```python
from build123d import *

# Parameters (mm, degrees)
SKETCH1_W           = 6.35
SKETCH1_H           = 3.0988
SKETCH1_H_2         = 25.146
BOSS_EXTRUDE1_DEPTH = 6.35


with BuildPart() as part:
    # Sketch1 → Boss-Extrude1 (new body)
    with BuildSketch(Plane(origin=(0, 0, -130.81), x_dir=(-1, 0, 0), z_dir=(0, 0, -1))):
        with BuildLine():
            Line((70.526798569, 59.314378099), (70.526798569, 62.413178099))
            Line((70.526798569, 62.413178099), (70.526798569, 81.336178099))
            ThreePointArc((70.526798569, 81.336178099), (63.856531257, 106.917123969), (45.544320246, 125.983853774))
            ThreePointArc((45.544320246, 125.983853774), (44.656455469, 126.90830128), (44.333048569, 128.148589564))
            Line((44.333048569, 128.148589564), (44.333048569, 147.869312576))
            ThreePointArc((44.333048569, 147.869312576), (43.589099793, 149.6653638), (41.793048569, 150.409312576))
            Line((41.793048569, 150.409312576), (-5.514451431, 150.409312576))
            ThreePointArc((-5.514451431, 150.409312576), (-7.310502655, 149.6653638), (-8.054451431, 147.869312576))
            Line((-8.054451431, 147.869312576), (-8.054451431, 128.668205083))
            ThreePointArc((-8.054451431, 128.668205083), (-8.464181451, 127.284893905), (-9.561183568, 126.347869434))
            Line((-9.561183568, 126.347869434), (-25.826658021, 119.104696647))
            Line((-25.826658021, 119.104696647), (-28.657467512, 117.844109854))
            Line((-28.657467512, 117.844109854), (-34.829560338, 115.095617339))
            Line((-34.829560338, 115.095617339), (-37.66036983, 113.835030546))
            Line((-37.66036983, 113.835030546), (-62.952028403, 102.57241084))
            Line((-62.952028403, 102.57241084), (-65.782837894, 101.311824047))
            Line((-65.782837894, 101.311824047), (-71.95493072, 98.563331532))
            Line((-71.95493072, 98.563331532), (-74.785740212, 97.302744739))
            Line((-74.785740212, 97.302744739), (-88.791116459, 91.0660155))
            ThreePointArc((-88.791116459, 91.0660155), (-105.234258555, 80.148597196), (-117.184308425, 64.439897298))
            ThreePointArc((-117.184308425, 64.439897298), (-118.119343883, 63.446350606), (-119.433558814, 63.079928099))
            Line((-119.433558814, 63.079928099), (-138.48728746, 63.079928099))
            ThreePointArc((-138.48728746, 63.079928099), (-140.283338684, 62.335979323), (-141.02728746, 60.539928099))
            Line((-141.02728746, 60.539928099), (-141.02728746, 13.232428099))
            ThreePointArc((-141.02728746, 13.232428099), (-140.283338684, 11.436376875), (-138.48728746, 10.692428099))
            Line((-138.48728746, 10.692428099), (-119.433558814, 10.692428099))
            ThreePointArc((-119.433558814, 10.692428099), (-118.119343883, 10.326005592), (-117.184308425, 9.3324589))
            ThreePointArc((-117.184308425, 9.3324589), (-105.234258555, -6.376240998), (-88.791116459, -17.293659302))
            Line((-88.791116459, -17.293659302), (-74.785740212, -23.530388541))
            Line((-74.785740212, -23.530388541), (-71.95493072, -24.790975333))
            Line((-71.95493072, -24.790975333), (-65.782837894, -27.539467849))
            Line((-65.782837894, -27.539467849), (-62.952028403, -28.800054642))
            Line((-62.952028403, -28.800054642), (-37.66036983, -40.062674348))
            Line((-37.66036983, -40.062674348), (-34.829560338, -41.323261141))
            Line((-34.829560338, -41.323261141), (-28.657467512, -44.071753656))
            Line((-28.657467512, -44.071753656), (-25.826658021, -45.332340449))
            Line((-25.826658021, -45.332340449), (-9.561183568, -52.575513236))
            ThreePointArc((-9.561183568, -52.575513236), (-8.464181451, -53.512537707), (-8.054451431, -54.895848885))
            Line((-8.054451431, -54.895848885), (-8.054451431, -76.636956378))
            Line((-8.054451431, -76.636956378), (44.333048569, -76.636956378))
            Line((44.333048569, -76.636956378), (44.333048569, -54.376233366))
            ThreePointArc((44.333048569, -54.376233366), (44.656455469, -53.135945082), (45.544320246, -52.211497576))
            ThreePointArc((45.544320246, -52.211497576), (63.856531257, -33.144767771), (70.526798569, -7.563821901))
            Line((70.526798569, -7.563821901), (70.526798569, 11.359178099))
            Line((70.526798569, 11.359178099), (70.526798569, 14.457978099))
            Line((70.526798569, 14.457978099), (70.526798569, 21.214378099))
            Line((70.526798569, 21.214378099), (70.526798569, 24.313178099))
            Line((70.526798569, 24.313178099), (70.526798569, 49.459178099))
            Line((70.526798569, 49.459178099), (70.526798569, 52.557978099))
            Line((70.526798569, 52.557978099), (70.526798569, 59.314378099))
        make_face()
        with Locations((73.701798569, 60.863778099)):
            Rectangle(SKETCH1_W, SKETCH1_H)
        with BuildLine():
            Line((70.526798569, 81.336178099), (70.526798569, 62.413178099))
            Line((70.526798569, 62.413178099), (76.876798569, 62.413178099))
            Line((76.876798569, 62.413178099), (76.876798569, 81.336178099))
            ThreePointArc((76.876798569, 81.336178099), (69.915897636, 109.072033869), (50.683048569, 130.234012838))
            Line((50.683048569, 130.234012838), (50.683048569, 154.219312576))
            ThreePointArc((50.683048569, 154.219312576), (49.939099793, 156.0153638), (48.143048569, 156.759312576))
            Line((48.143048569, 156.759312576), (-11.864451431, 156.759312576))
            ThreePointArc((-11.864451431, 156.759312576), (-13.660502655, 156.0153638), (-14.404451431, 154.219312576))
            Line((-14.404451431, 154.219312576), (-14.404451431, 131.142265008))
            Line((-14.404451431, 131.142265008), (-28.409827678, 124.905535769))
            Line((-28.409827678, 124.905535769), (-25.826658021, 119.104696647))
            Line((-25.826658021, 119.104696647), (-9.561183568, 126.347869434))
            ThreePointArc((-9.561183568, 126.347869434), (-8.464181451, 127.284893905), (-8.054451431, 128.668205083))
            Line((-8.054451431, 128.668205083), (-8.054451431, 147.869312576))
            ThreePointArc((-8.054451431, 147.869312576), (-7.310502655, 149.6653638), (-5.514451431, 150.409312576))
            Line((-5.514451431, 150.409312576), (41.793048569, 150.409312576))
            ThreePointArc((41.793048569, 150.409312576), (43.589099793, 149.6653638), (44.333048569, 147.869312576))
            Line((44.333048569, 147.869312576), (44.333048569, 128.148589564))
            ThreePointArc((44.333048569, 128.148589564), (44.656455469, 126.90830128), (45.544320246, 125.983853774))
            ThreePointArc((45.544320246, 125.983853774), (63.856531257, 106.917123969), (70.526798569, 81.336178099))
        make_face()
        with Locations((73.701798569, 51.008578099)):
            Rectangle(SKETCH1_W, SKETCH1_H)
        with Locations((73.701798569, 36.886178099)):
            Rectangle(SKETCH1_W, SKETCH1_H_2)
        with Locations((73.701798569, 22.763778099)):
            Rectangle(SKETCH1_W, SKETCH1_H)
        with Locations((73.701798569, 12.908578099)):
            Rectangle(SKETCH1_W, SKETCH1_H)
        with BuildLine():
            Line((76.876798569, 11.359178099), (70.526798569, 11.359178099))
            Line((70.526798569, 11.359178099), (70.526798569, -7.563821901))
            ThreePointArc((70.526798569, -7.563821901), (63.856531257, -33.144767771), (45.544320246, -52.211497576))
            ThreePointArc((45.544320246, -52.211497576), (44.656455469, -53.135945082), (44.333048569, -54.376233366))
            Line((44.333048569, -54.376233366), (44.333048569, -76.636956378))
            Line((44.333048569, -76.636956378), (-8.054451431, -76.636956378))
            Line((-8.054451431, -76.636956378), (-8.054451431, -54.895848885))
            ThreePointArc((-8.054451431, -54.895848885), (-8.464181451, -53.512537707), (-9.561183568, -52.575513236))
            Line((-9.561183568, -52.575513236), (-25.826658021, -45.332340449))
            Line((-25.826658021, -45.332340449), (-28.409827678, -51.133179571))
            Line((-28.409827678, -51.133179571), (-14.404451431, -57.36990881))
            Line((-14.404451431, -57.36990881), (-14.404451431, -80.446956378))
            ThreePointArc((-14.404451431, -80.446956378), (-13.660502655, -82.243007602), (-11.864451431, -82.986956378))
            Line((-11.864451431, -82.986956378), (48.143048569, -82.986956378))
            ThreePointArc((48.143048569, -82.986956378), (49.939099793, -82.243007602), (50.683048569, -80.446956378))
            Line((50.683048569, -80.446956378), (50.683048569, -56.46165664))
            ThreePointArc((50.683048569, -56.46165664), (69.915897636, -35.299677671), (76.876798569, -7.563821901))
            Line((76.876798569, -7.563821901), (76.876798569, 11.359178099))
        make_face()
        Polygon((-28.409827678, -51.133179571), (-25.826658021, -45.332340449), (-28.657467512, -44.071753656), (-31.24063717, -49.872592778), align=None)
        Polygon((-37.412729996, -47.124100263), (-34.829560338, -41.323261141), (-37.66036983, -40.062674348), (-40.243539487, -45.86351347), align=None)
        Polygon((-40.243539487, -45.86351347), (-37.66036983, -40.062674348), (-62.952028403, -28.800054642), (-65.53519806, -34.600893764), align=None)
        Polygon((-65.53519806, -34.600893764), (-62.952028403, -28.800054642), (-65.782837894, -27.539467849), (-68.366007552, -33.340306971), align=None)
        with BuildLine():
            Line((-74.785740212, 97.302744739), (-77.368909869, 103.103583861))
            Line((-77.368909869, 103.103583861), (-91.374286117, 96.866854622))
            ThreePointArc((-91.374286117, 96.866854622), (-108.722690302, 85.568449718), (-121.690697129, 69.429928099))
            Line((-121.690697129, 69.429928099), (-144.83728746, 69.429928099))
            ThreePointArc((-144.83728746, 69.429928099), (-146.633338684, 68.685979323), (-147.37728746, 66.889928099))
            Line((-147.37728746, 66.889928099), (-147.37728746, 6.882428099))
            ThreePointArc((-147.37728746, 6.882428099), (-146.633338684, 5.086376875), (-144.83728746, 4.342428099))
            Line((-144.83728746, 4.342428099), (-121.690697129, 4.342428099))
            ThreePointArc((-121.690697129, 4.342428099), (-108.722690302, -11.79609352), (-91.374286117, -23.094498424))
            Line((-91.374286117, -23.094498424), (-77.368909869, -29.331227663))
            Line((-77.368909869, -29.331227663), (-74.785740212, -23.530388541))
            Line((-74.785740212, -23.530388541), (-88.791116459, -17.293659302))
            ThreePointArc((-88.791116459, -17.293659302), (-105.234258555, -6.376240998), (-117.184308425, 9.3324589))
            ThreePointArc((-117.184308425, 9.3324589), (-118.119343883, 10.326005592), (-119.433558814, 10.692428099))
            Line((-119.433558814, 10.692428099), (-138.48728746, 10.692428099))
            ThreePointArc((-138.48728746, 10.692428099), (-140.283338684, 11.436376875), (-141.02728746, 13.232428099))
            Line((-141.02728746, 13.232428099), (-141.02728746, 60.539928099))
            ThreePointArc((-141.02728746, 60.539928099), (-140.283338684, 62.335979323), (-138.48728746, 63.079928099))
            Line((-138.48728746, 63.079928099), (-119.433558814, 63.079928099))
            ThreePointArc((-119.433558814, 63.079928099), (-118.119343883, 63.446350606), (-117.184308425, 64.439897298))
            ThreePointArc((-117.184308425, 64.439897298), (-105.234258555, 80.148597196), (-88.791116459, 91.0660155))
            Line((-88.791116459, 91.0660155), (-74.785740212, 97.302744739))
        make_face()
        Polygon((-74.538100378, -30.591814456), (-71.95493072, -24.790975333), (-74.785740212, -23.530388541), (-77.368909869, -29.331227663), align=None)
        Polygon((-37.66036983, 113.835030546), (-40.243539487, 119.635869668), (-65.53519806, 108.373249962), (-62.952028403, 102.57241084), align=None)
        Polygon((-34.829560338, 115.095617339), (-37.412729996, 120.896456461), (-40.243539487, 119.635869668), (-37.66036983, 113.835030546), align=None)
        Polygon((-25.826658021, 119.104696647), (-28.409827678, 124.905535769), (-31.24063717, 123.644948976), (-28.657467512, 117.844109854), align=None)
        Polygon((-62.952028403, 102.57241084), (-65.53519806, 108.373249962), (-68.366007552, 107.112663169), (-65.782837894, 101.311824047), align=None)
        Polygon((-71.95493072, 98.563331532), (-74.538100378, 104.364170654), (-77.368909869, 103.103583861), (-74.785740212, 97.302744739), align=None)
    extrude(amount=BOSS_EXTRUDE1_DEPTH)


solid = part.part
```
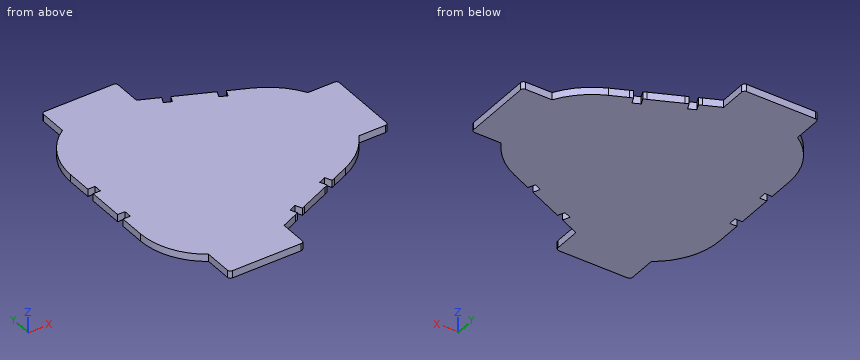
Could you check a few things on this model? Use its own coordinates, in mm. Give positions to 0.01 mm unless a question says otherwise; leave off trailing zeros. Loops run counter-clockwise (first coordinate to the right, second up) from the corner with the lowest first, then second, coordinate; pieces in that order, holes last. Notation, with made-up numbers: (68.25, 18) - (96.25, 18) arc R9 ccw to (96.25, 34) - close; hole circle Ø7 at (-18.5, 43). An arc over 180 degrees is marked (long way). Answer in a Markdown table with one row per item. Add a question column.
Q1. If we section it at B-B (x = 96.5): List the corners of the cut face in (y, z) for me, plus the area to 3 significant figures.
Q2. If we section it at A-A (y = -64.5): List the corners of the cut face in (x, z) for me, plus the area to 3 significant figures.
Q3. For pin 1 (3 mm diameter, centred on x = 132, z = -135.5, fed in from -Y); pin 2 (3 mm diameter, centred on y = 141.5, z = -133.5, fed in from -X); pin 3 (1.9 mm diameter, centred on y = 144.5, z = -132.5, fed in from +X), each with a flat end and sliding along its axis, tell me the tip position at first contact or that it passes through.
Q4. Please list where these lines run through material, in increasing order: L1, parallel to X at y = -73, z = -135.5; L2, parallel to Y at x = 29.5, z = -135; L3, parallel to Y at x = 126.5, z = -136. Write a range as from..to.
The answers:
| question | item | result |
|---|---|---|
| 1 | outline | (-20.54, -137.16) - (94.31, -137.16) - (94.31, -130.81) - (-20.54, -130.81) - close |
| 1 | area | 729 mm^2 |
| 2 | outline | (-50.68, -137.16) - (14.4, -137.16) - (14.4, -130.81) - (-50.68, -130.81) - close |
| 2 | area | 413 mm^2 |
| 3 | pin 1 | stops at y = 4.34 |
| 3 | pin 2 | stops at x = -50.68 |
| 3 | pin 3 | stops at x = 14.4 |
| 4 | L1 | x = -50.68..14.4 |
| 4 | L2 | y = -50.65..-45.96, -43.7..117.47, 119.74..124.42 |
| 4 | L3 | y = 4.34..69.43 |
